Could you check a few things on this drawing? It's one solid part, dimensions in mm from its lowest x, y, z. Give positions to 0.01 mm unless a question says otherwise; leave off trailing zeros. Loops run counter-clockwise (first coordinate to the right, second up) from the corner with the lowest first, then second, coordinate; pieces in that order, holes last. Notation, with made-up numbers: M 55,69.5 L 88,69.5 A6 ccw 88,74.5 Z; hole C -30.75,73 d1. An arc over 180 degrees is marked long. Answer as CSV lines item,"result". Start each with the question number.
Item 1: I want a section at A-A on x = 40. List the corners of the cut face in (y, z) for me (1 decimal).
Item 2: If I drill on line 1 along Y through (x, z) = (40, 1.2) (1 decimal); line 2 along Y through (x, z) = (34, 0.45) (1 decimal); line 3 along Y through (x, z) = (42.14, 0.95) (1 decimal), over which ranges is the centre line in solid material (lowest first)? Write a range as from..to.
Item 3: I want a section at C-C on x = 32.14. List the corners of the cut face in (y, z) for me (1 decimal).
Item 4: I want a section at B-B on y = 10. List the corners of the cut face in (x, z) for me.
Item 5: I want a section at D-D on z = 0.5. List the corners of the cut face in (x, y) for me (1 decimal), plus the area to 3 significant figures.
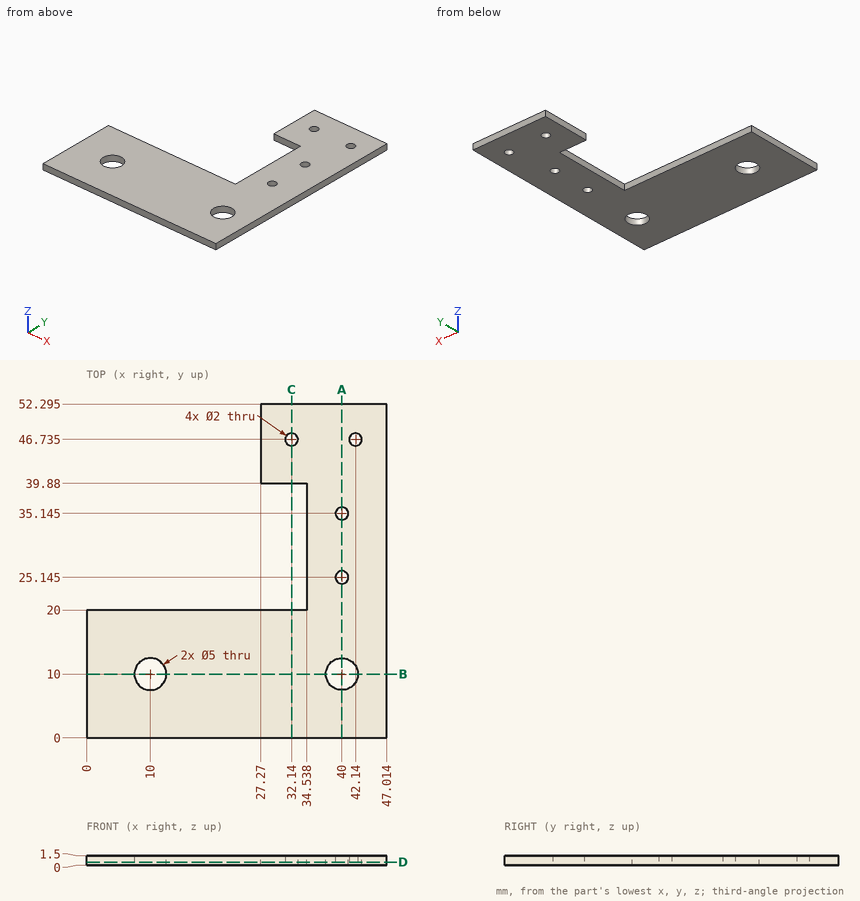
Result:
1,outline,"M 0,0 L 7.5,0 L 7.5,1.5 L 0,1.5 Z; M 12.5,0 L 24.1,0 L 24.1,1.5 L 12.5,1.5 Z; M 26.1,0 L 34.1,0 L 34.1,1.5 L 26.1,1.5 Z; M 36.1,0 L 52.3,0 L 52.3,1.5 L 36.1,1.5 Z"
2,line 1,"0..7.5, 12.5..24.1, 26.1..34.1, 36.1..52.3"
2,line 2,"0..20, 39.9..52.3"
2,line 3,"0..8.7, 11.3..45.7, 47.7..52.3"
3,outline,"M 0,0 L 20,0 L 20,1.5 L 0,1.5 Z; M 39.9,0 L 45.7,0 L 45.7,1.5 L 39.9,1.5 Z; M 47.7,0 L 52.3,0 L 52.3,1.5 L 47.7,1.5 Z"
4,outline,"M 0,0 L 7.5,0 L 7.5,1.5 L 0,1.5 Z; M 12.5,0 L 37.5,0 L 37.5,1.5 L 12.5,1.5 Z; M 42.5,0 L 47.01,0 L 47.01,1.5 L 42.5,1.5 Z"
5,outline,"M 0,0 L 47,0 L 47,52.3 L 27.3,52.3 L 27.3,39.9 L 34.5,39.9 L 34.5,20 L 0,20 Z; hole C 10,10 d5; hole C 32.1,46.7 d2; hole C 40,10 d5; hole C 40,25.1 d2; hole C 40,35.1 d2; hole C 42.1,46.7 d2"
5,area,"1,380 mm^2"
